Source: CAD feature listing. Evaluate the final solid. Frame: model axes, mm. Coordinates: 2 decimals unless noted, no trailing zeros. Loops run counter-clockwise (first coordinate to the right, second up) from the corner with the lowest first, then second, coordinate; pieces in that order, holes last.
```python
from build123d import *

# Parameters (mm, degrees)
SKETCH1_W           = 20
SKETCH1_H           = 20
SKETCH1_R           = 4
BOSS_EXTRUDE1_DEPTH = 10
SKETCH2_R           = 1.15
SKETCH2_R_2         = 2.1
CUT_EXTRUDE1_DEPTH  = 21
CHAMFER1_SIZE       = 5


with BuildPart() as part:
    # Sketch1 → Boss-Extrude1 (new body)
    with BuildSketch(Plane.XY):
        with Locations((10, 10)):
            Rectangle(SKETCH1_W, SKETCH1_H)
        with Locations((10, 10)):
            Circle(SKETCH1_R, mode=Mode.SUBTRACT)
    extrude(amount=BOSS_EXTRUDE1_DEPTH)

    # Sketch2 → Cut-Extrude1 (cut, through all)
    with BuildSketch(Plane(origin=(0, 20, 0), x_dir=(1, 0, 0), z_dir=(0, 1, 0))):
        with Locations((3, -7)):
            Circle(SKETCH2_R)
        with Locations((17, -3)):
            Circle(SKETCH2_R)
        with Locations((10, -5)):
            Circle(SKETCH2_R_2)
    extrude(amount=-CUT_EXTRUDE1_DEPTH, mode=Mode.SUBTRACT)

    # Chamfer1
    chamfer1_edges = [part.edges().sort_by_distance(p)[0] for p in [
        (0, 10, 0),
    ]]
    chamfer(chamfer1_edges, length=CHAMFER1_SIZE)


solid = part.part
```
Q1. Section query C-C on x = 17. Return the cut outline in (y, z).
Q2. Section query D-D on z = 2.5. Return the cut outline in (x, y).
Q3. Section query A-A on x = 10. Return the cut outline in (y, z).
Q4. Section query B-B on y = 10. Return the cut outline in (x, z).
Q5. Material intervals for line 1 along X through (y, z) = (9.5, 7); line 2 along X through (y, z) = (16.5, 3.5); line 3 along Z through (x, y) = (10, 15.5), sorted ascending.
Q6. Draft query along Z for faces 1 (the flat face through (20, 10, 5)), 2 (the flat face through (3, 10, 2)), 3 (the cylindrical face through (7.9, 3.34, 4.91)). Return one class per face: released by +Z, released by -Z, zero draft, split by the parting line, or undercut.
Q7. First-contact query: pin 1 Ø4 at (y, z) = (15.5, 2) entering from -X. Flat tip, straight axial feed; report the tip coordinate or a pass-through.
Resolved:
1. outline: (0, 0) - (20, 0) - (20, 1.85) - (0, 1.85) - close; (0, 4.15) - (20, 4.15) - (20, 10) - (0, 10) - close
2. outline: (2.5, 0) - (15.96, 0) - (15.96, 20) - (2.5, 20) - close; (18.04, 0) - (20, 0) - (20, 20) - (18.04, 20) - close; hole circle Ø8 at (10, 10)
3. outline: (0, 0) - (6, 0) - (6, 2.9) - (0, 2.9) - close; (0, 7.1) - (6, 7.1) - (6, 10) - (0, 10) - close; (14, 0) - (20, 0) - (20, 2.9) - (14, 2.9) - close; (14, 7.1) - (20, 7.1) - (20, 10) - (14, 10) - close
4. outline: (0, 5) - (5, 0) - (6, 0) - (6, 10) - (0, 10) - close; (14, 0) - (20, 0) - (20, 10) - (14, 10) - close; hole circle Ø2.3 at (3, 7); hole circle Ø2.3 at (17, 3)
5. line 1: x = 0 to 1.85, 4.15 to 6.03, 13.97 to 20
5. line 2: x = 1.5 to 8.53, 11.47 to 15.96, 18.04 to 20
5. line 3: z = 0 to 2.9, 7.1 to 10
6. face 1: zero draft
6. face 2: released by -Z
6. face 3: undercut
7. pin 1: stops at x = 1
